Autodesk Inventor part; units mm, degrees
ref_plane "YZ Plane" through (0, 0, 0) normal (1, 0, 0) x (0, 1, 0)
ref_plane "XZ Plane" through (0, 0, 0) normal (0, 1, 0) x (-1, 0, 0)
ref_plane "XY Plane" through (0, 0, 0) normal (0, 0, 1) x (1, 0, 0)
sketch "Skizze5" plane through (0, 0, 0) normal (0, 0, 1) x (1, 0, 0)
  line L0 (-8.1928, -13.75) -> (8.1928, -13.75)
  arc A0 (13.75, -8.1928) -> (8.1928, -13.75) centre (11.5, -11.5) ccw
  line L1 (13.75, -8.1928) -> (13.75, 8.1928)
  arc A1 (8.1928, 13.75) -> (13.75, 8.1928) centre (11.5, 11.5) ccw
  line L2 (8.1928, 13.75) -> (-8.1928, 13.75)
  arc A2 (-13.75, 8.1928) -> (-8.1928, 13.75) centre (-11.5, 11.5) ccw
  line L3 (-13.75, 8.1928) -> (-13.75, -8.1928)
  arc A3 (-8.1928, -13.75) -> (-13.75, -8.1928) centre (-11.5, -11.5) ccw
  circle A4 centre (0, 0) radius 4
  circle A5 centre (0, 0) radius 2.2643 construction
  circle A6 centre (0, 10.9602) radius 2 construction
  circle A7 centre (0, -10.9602) radius 2 construction
  circle A8 centre (10.9602, 0) radius 2 construction
  circle A9 centre (-10.9602, 0) radius 2 construction
  line L4 (13.0815, -2.8284) -> (2.8284, -13.0815) construction
  arc A10 (13.0815, -2.8284) -> (13.0815, 2.8284) centre (10.253, 0) ccw construction
  line L5 (2.8284, 13.0815) -> (13.0815, 2.8284) construction
  arc A11 (2.8284, 13.0815) -> (-2.8284, 13.0815) centre (0, 10.253) ccw construction
  line L6 (-13.0815, 2.8284) -> (-2.8284, 13.0815) construction
  arc A12 (-13.0815, 2.8284) -> (-13.0815, -2.8284) centre (-10.253, 0) ccw construction
  line L7 (-2.8284, -13.0815) -> (-13.0815, -2.8284) construction
  arc A13 (-2.8284, -13.0815) -> (2.8284, -13.0815) centre (0, -10.253) ccw construction
  arc A14 (14.25, 12.25) -> (12.25, 14.25) centre (12.25, 12.25) ccw construction
  arc A15 (-14.25, -12.25) -> (-12.25, -14.25) centre (-12.25, -12.25) ccw construction
  line L8 (-14.25, -14.25) -> (14.25, -14.25)
  line L9 (14.25, -14.25) -> (14.25, 14.25)
  line L10 (14.25, 14.25) -> (-14.25, 14.25)
  line L11 (-14.25, 14.25) -> (-14.25, -14.25)
  line L12 (-14.25, -14.25) -> (14.25, 14.25) construction
  line L13 (14.25, -14.25) -> (-14.25, 14.25) construction
  circle A16 centre (10.9602, 0) radius 1.4
  circle A17 centre (0, 10.9602) radius 1.4
  circle A18 centre (0, -10.9602) radius 1.4
  circle A19 centre (-10.9602, 0) radius 1.4
  line L14 (-11.1369, 4.773) -> (4.773, -11.1369)
  line L15 (4.773, -11.1369) -> (11.1369, -4.773)
  line L16 (11.1369, -4.773) -> (-4.773, 11.1369)
  line L17 (-4.773, 11.1369) -> (-11.1369, 4.773)
  line L18 (-11.1369, 4.773) -> (11.1369, -4.773) construction
  line L19 (4.773, -11.1369) -> (-4.773, 11.1369) construction
  line L20 (11.1369, 4.773) -> (-4.773, -11.1369)
  line L21 (-4.773, -11.1369) -> (-11.1369, -4.773)
  line L22 (-11.1369, -4.773) -> (4.773, 11.1369)
  line L23 (4.773, 11.1369) -> (11.1369, 4.773)
  line L24 (11.1369, 4.773) -> (-11.1369, -4.773) construction
  line L25 (-4.773, -11.1369) -> (4.773, 11.1369) construction
  circle A20 centre (11.5, 11.5) radius 1.4
  circle A21 centre (11.5, -11.5) radius 1.4
  circle A22 centre (-11.5, -11.5) radius 1.4
  circle A23 centre (-11.5, 11.5) radius 1.4
  point P0 (0, 0)
  point P1 (0, -6.364)
  point P2 (-6.364, 0)
  point P3 (0, 6.364)
  point P4 (6.364, 0)
  dimension "d13" = 2.8
  dimension "d14" = 2.8
  dimension "d15" = 2.8
  dimension "d16" = 2.8
  dimension "d17" = 9
  dimension "d18" = 9
extrude "Extrusion4" add sketch "Skizze5" along normal blind 4.5 contours A3 L3 A2 L2 A1 L1 A0 L0 | L11 L10 L9 L8
fillet "Rundung2" radius 2 16 edges at (14.25, 14.25, 2.25) (14.25, -14.25, 2.25) (-14.25, -14.25, 2.25) (-14.25, 14.25, 2.25) (0, 6.364, 2.25) (4.773, 11.1369, 2.25) (-4.773, 11.1369, 2.25) (-11.1369, 4.773, 2.25) (-6.364, 0, 2.25) (-11.1369, -4.773, 2.25) (-4.773, -11.1369, 2.25) (0, -6.364, 2.25) (4.773, -11.1369, 2.25) (11.1369, -4.773, 2.25) (6.364, 0, 2.25) (11.1369, 4.773, 2.25)
sketch "Skizze6" plane through (0, 0, 0) normal (0, 0, -1) x (-1, 0, 0)
  line L0 (-14.25, -12.25) -> (-14.25, -8.1928)
  arc A0 (-14.25, -8.1928) -> (-13.4687, -8.6062) centre (-13.75, -8.1928) ccw
  arc A1 (-8.6062, -13.4688) -> (-13.4687, -8.6062) centre (-11.5, -11.5) ccw
  arc A2 (-8.6062, -13.4688) -> (-8.1928, -14.25) centre (-8.1928, -13.75) ccw
  line L1 (-8.1928, -14.25) -> (-12.25, -14.25)
  arc A3 (-14.25, -12.25) -> (-12.25, -14.25) centre (-12.25, -12.25) ccw
  circle A4 centre (-11.5, -11.5) radius 1.4
  line L2 (8.1928, 14.25) -> (12.25, 14.25)
  arc A5 (14.25, 12.25) -> (12.25, 14.25) centre (12.25, 12.25) ccw
  line L3 (14.25, 12.25) -> (14.25, 8.1928)
  arc A6 (14.25, 8.1928) -> (13.4688, 8.6062) centre (13.75, 8.1928) ccw
  arc A7 (8.6062, 13.4688) -> (13.4688, 8.6062) centre (11.5, 11.5) ccw
  arc A8 (8.6062, 13.4688) -> (8.1928, 14.25) centre (8.1928, 13.75) ccw
  circle A9 centre (11.5, 11.5) radius 1.4
  point P0 (0, 0)
extrude "Extrusion5" [suppressed]
properties part number "30_Adapter_AS5600_rotational_enocder_nema12"
Can you work these out from the model? Positions are in its coordinate system, mm. A direction names the side the tool comes from. Give positions to 0.01 mm unless a question says otherwise; leave off trailing zeros. Order: outer loops, then holes, each group sorted by start corner. A loop starts at its lowest first (then second) coordinate and runs counter-clockwise, first axis right, second up. Notation, with made-up numbers: M 77,69 L 130,69 A17 cw 130,82 Z; hole C 65.25,-2.5 d5. An arc over 180 degrees is marked long. Use a Markdown table: item, result. Add a question column.
Item 1: Suppose I cut it at B-B (y = -11.5). List the corners of the cut face in (x, z) for me, then the cut area to 3 significant figures.
Item 2: Suppose I cut it at D-D (y = -4.5). List the corners of the cut face in (x, z) for me.
Item 3: For faces 1 (the flat face through (3, 10, 4.5)), 2 (the flat face through (-8.764, -2.4, 2.218)), which set-ups out of +Z, -Z, +X, -X, +Y, -Y let a thin tool reach every point of the face, with its end or its side?
Item 4: If I drill on L1, parallel to Y at x = 0, z = 3.5; L2, parallel to X at y = 0.25, z = 0.3; L3, parallel to Y at x = 11.5, z = 2.45, over which ranges is the centre line in solid material (lowest first)? Write a range as [from, to].
Item 5: We'd pull the mould along X, two halves only. Please class faces 3 (the cylindrical face through (-13.65, 13.68, 2.28)), 4 (the flat face through (3, 10, 0)), 5 (the cylindrical face through (10.47, -12.45, 2.22)): +X half, -X half, draft (parallel to the pull), parting line (faces both ways), or undercut.
Item 6: Suppose I cut it at C-C (x = -5.5). List the corners of the cut face in (y, z) for me, then the cut area to 3 significant figures.
Item 7: Suppose I cut it at A-A (x = 0). List the corners of the cut face in (y, z) for me.
Answer sheet:
| question | item | result |
|---|---|---|
| 1 | outline | M -14.25,0 L -12.9,0 L -12.9,4.5 L -14.25,4.5 Z; M -10.1,0 L -1.29,0 L -1.29,4.5 L -10.1,4.5 Z; M 1.29,0 L 10.1,0 L 10.1,4.5 L 1.29,4.5 Z; M 12.9,0 L 14.25,0 L 14.25,4.5 L 12.9,4.5 Z |
| 1 | area | 91.4 mm² |
| 2 | outline | M -14.25,0 L -10.29,0 L -10.29,4.5 L -14.25,4.5 Z; M 10.29,0 L 14.25,0 L 14.25,4.5 L 10.29,4.5 Z |
| 3 | face 1 | +Z, +X, -X, +Y, -Y |
| 3 | face 2 | +Z, -Z |
| 4 | L1 | y = [-14.25, -12.36], [-9.56, -7.19], [7.19, 9.56], [12.36, 14.25] |
| 4 | L2 | x = [-14.25, -12.34], [-9.58, -7.21], [7.21, 9.58], [12.34, 14.25] |
| 4 | L3 | y = [-14.25, -12.9], [-10.1, -1.29], [1.29, 10.1], [12.9, 14.25] |
| 5 | face 3 | -X half |
| 5 | face 4 | draft |
| 5 | face 5 | undercut |
| 6 | outline | M -14.25,0 L -10.17,0 L -10.17,4.5 L -14.25,4.5 Z; M 10.17,0 L 14.25,0 L 14.25,4.5 L 10.17,4.5 Z |
| 6 | area | 36.7 mm² |
| 7 | outline | M -14.25,0 L -12.36,0 L -12.36,4.5 L -14.25,4.5 Z; M -9.56,0 L -7.19,0 L -7.19,4.5 L -9.56,4.5 Z; M 7.19,0 L 9.56,0 L 9.56,4.5 L 7.19,4.5 Z; M 12.36,0 L 14.25,0 L 14.25,4.5 L 12.36,4.5 Z |
